Work out the finished part from the listing and answer in its coordinate system (mm). Face numbers are marked on the shaded views. A direction names the side the tool comes from. Give positions to 0.01 mm unless a question says otherwise; leave off trailing zeros. Order: outer loops, then holes, each group sorted by start corner. A loop starts at its lowest first (then second) coordinate and runs counter-clockwise, first axis right, second up. Notation, with made-up numbers: M 52.5,-16.5 L 63.5,-16.5 A29 cw 63.5,19.5 Z; hole C 3,35.25 d5. An arc over 180 degrees is marked long. One line per item, written item: value.
Solid Edge part; units mm, degrees
sketch "Sketch1" plane through (0, 0, 0) normal (0, -1, 0) x (1, 0, 0)
  line L0 (31.4924, 49.0939) -> (121.4924, 49.0939)
  line L1 (121.4924, 49.0939) -> (121.4924, 9.0939)
  line L2 (121.4924, 9.0939) -> (31.4924, 9.0939)
  line L3 (31.4924, 9.0939) -> (31.4924, 49.0939)
  dimension "D1" = 31.4924
  dimension "D2" = 121.4924
extrude "Protrusion1" add sketch "Sketch1" against normal blind 40
sketch "Sketch2" plane through (64.4924, 0, 22.0939) normal (0, -1, 0) x (1, 0, 0)
  line L0 (-18.0616, 9.8803) -> (-8, 10.7605)
  line L1 (-8, 10.7605) -> (-8, 18.0605)
  line L2 (-8, 18.0605) -> (34, 18.0605)
  line L3 (34, -4) -> (34, 18.0605)
  line L4 (-8, -4) -> (34, -4)
  line L5 (-8, -4) -> (-8, 3.3)
  line L6 (-8, 3.3) -> (-18.0616, 4.1803)
  line L7 (-18.0616, 4.1803) -> (-18.0616, 9.8803)
extrude "ExtrudedCutout_4" cut sketch "Sketch2" against normal blind 37
sketch "Sketch3" plane through (31.4924, 20, 22.0939) normal (-1, 0, 0) x (0, -1, 0)
  line L0 (-17, 2) -> (-17, 12)
  line L1 (-17, 12) -> (-10, 12)
  line L2 (-10, 12) -> (-10, 2)
  line L3 (-10, 2) -> (-17, 2)
  dimension "D1" = 17
  dimension "D2" = 17
  dimension "D3" = 10
extrude "Cutout1" cut sketch "Sketch3" against normal up to next
sketch "Sketch4" plane through (64.4924, 0, 22.0939) normal (0, -1, 0) x (1, 0, 0)
  line L0 (-8, 17.0605) -> (-18, 17.0605)
  line L1 (-18, 17.0605) -> (-18, -2.9395)
  line L2 (-18, -2.9395) -> (-8, -2.9395)
  line L3 (-8, -2.9395) -> (-8, 17.0605)
  line L4 (34, 17.0605) -> (44, 17.0605)
  line L5 (44, 17.0605) -> (44, -2.9395)
  line L6 (44, -2.9395) -> (34, -2.9395)
  line L7 (34, -2.9395) -> (34, 17.0605)
  dimension "D1" = 44
  dimension "D2" = 8
  dimension "D3" = 18
  dimension "D4" = 34
extrude "ExtrudedCutout_6" cut sketch "Sketch4" against normal blind 10
sketch "Sketch5" plane through (91.2324, 10, 21.645) normal (0, -1, 0) x (1, 0, 0)
  circle A0 centre (11.76, 12.5095) radius 1.65
  circle A1 centre (-39.24, 12.5095) radius 1.65
  circle A2 centre (-39.24, 2.5095) radius 1.65
  circle A3 centre (11.76, 2.5095) radius 1.65
  dimension "D1" = 39.24
  dimension "D2" = 11.76
  dimension "D3" = 39.24
extrude "Cutout2" cut sketch "Sketch5" against normal through all
sketch "Sketch6" plane through (68.9924, 0, 22.0939) normal (0, -1, 0) x (1, 0, 0)
  line L0 (-37.5, 27) -> (-37.5, -13)
  line L1 (-37.5, -13) -> (52.5, -13)
  line L2 (52.5, -13) -> (52.5, 27)
  line L3 (52.5, 27) -> (-37.5, 27)
  line L4 (-22.5616, 13.0605) -> (-22.5616, 18.0605)
  line L5 (-22.5616, 18.0605) -> (39.5, 18.0605)
  line L6 (39.5, 18.0605) -> (39.5, -4)
  line L7 (39.5, -4) -> (-22.5616, -4)
  line L8 (-22.5616, 13.0605) -> (-22.5616, -4)
  dimension "D1" = 39.5
extrude "ExtrudedProtrusion_4" add sketch "Sketch6" along normal blind 28.07
sketch "Sketch7" plane through (68.9924, -28.07, 22.0939) normal (0, -1, 0) x (1, 0, 0)
  circle A0 centre (-4.46, 7) radius 23.5
extrude "ExtrudedCutout_9" cut sketch "Sketch7" against normal blind 33.07
sketch "Sketch8" plane through (41.8429, -28.07, 29.0939) normal (0, -1, 0) x (0, 0, 1)
  line L0 (0, 10.3505) -> (5, 10.3505)
  line L1 (5, 10.3505) -> (5, -79.6495)
  line L2 (5, -79.6495) -> (0, -79.6495)
  line L3 (0, -79.6495) -> (-5, -79.6495)
  line L4 (-5, -79.6495) -> (-5, 10.3505)
  line L5 (-5, 10.3505) -> (0, 10.3505)
  dimension "D1" = 5
extrude "Cutout3" cut sketch "Sketch8" against normal blind 15
sketch "Sketch9" plane through (76.4924, 5.965, 49.0939) normal (0, 0, 1) x (-1, 0, 0)
  line L0 (-0.379, 0.965) -> (24.299, 0.965)
  line L1 (24.299, 0.965) -> (45, 0.965)
  line L2 (45, 0.965) -> (55, 0.965)
  line L3 (55, 0.965) -> (55, -9.035)
  line L4 (55, -9.035) -> (45, -9.035)
  line L5 (45, -9.035) -> (-45, -9.035)
  line L6 (-45, -9.035) -> (-55, -9.035)
  line L7 (-55, -9.035) -> (-55, 0.965)
  line L8 (-55, 0.965) -> (-45, 0.965)
  line L9 (-45, 0.965) -> (-0.379, 0.965)
  dimension "D1" = 55
  dimension "D2" = 45
  dimension "D3" = 45
  dimension "D4" = 55
extrude "ExtrudedProtrusion_9" add sketch "Sketch9" against normal blind 8
sketch "Sketch10" plane through (26.4924, 10, 41.0939) normal (0, 0, -1) x (-1, 0, 0)
  circle A0 centre (0, 0) radius 2
  circle A1 centre (-100, 0) radius 2
extrude "Cutout4" cut sketch "Sketch10" against normal through all
chamfer "Chamfer_1" distance 10 angle 45 1 edges at (31.4924, 15, 45.0939)
chamfer "Chamfer_2" distance 10 angle 45 1 edges at (31.4924, 5, 45.0939)
chamfer "Chamfer_3" distance 10 angle 45 1 edges at (121.4924, 15, 45.0939)
chamfer "Chamfer_4" distance 10 angle 45 1 edges at (121.4924, 5, 45.0939)
sketch "Sketch11" plane through (76.4924, 5.965, 49.0939) normal (0, 0, 1) x (1, 0, 0)
  line L0 (-55, 9.035) -> (55, 9.035)
  line L1 (55, 9.035) -> (45, 34.035)
  line L2 (45, 34.035) -> (-45, 34.035)
  line L3 (-45, 34.035) -> (-55, 9.035)
extrude "Cutout5" cut sketch "Sketch11" against normal through all
sketch "Sketch12" plane through (99.1819, -28.07, 41.5939) normal (0, -1, 0) x (1, 0, 0)
  line L0 (-58.1495, -12.5) -> (-58.1495, 7.5)
  line L1 (-58.1495, 7.5) -> (0, 7.5)
  line L2 (0, 7.5) -> (9.3829, 7.5)
  line L3 (9.3829, 7.5) -> (9.3829, -32.5)
  line L4 (-58.1495, -32.5) -> (9.3829, -32.5)
  line L5 (-58.1495, -12.5) -> (-58.1495, -32.5)
extrude "Cutout6" cut sketch "Sketch12" against normal up to vertex (33.07 mm away)
sketch "Sketch13" plane through (36.2624, -28.07, 41.5939) normal (0, -1, 0) x (0, 0, -1)
  line L0 (2.5, -4.77) -> (2.5, 4.77)
  line L1 (2.5, 4.77) -> (7.5, 4.77)
  line L2 (7.5, 4.77) -> (7.5, -4.77)
  line L3 (7.5, -4.77) -> (2.5, -4.77)
extrude "Cutout7" cut sketch "Sketch13" against normal up to vertex (15 mm away)
sketch "Sketch14" plane through (36.2624, -28.07, 41.5939) normal (0, -1, 0) x (0, 0, -1)
  line L0 (22.5, 4.77) -> (22.5, -4.77)
  line L1 (22.5, -4.77) -> (17.5, -4.77)
  line L2 (17.5, -4.77) -> (17.5, 4.77)
  line L3 (17.5, 4.77) -> (22.5, 4.77)
extrude "Cutout8" cut sketch "Sketch14" against normal up to vertex (15 mm away)
sketch "Sketch15" plane through (36.2624, -28.07, 41.5939) normal (0, -1, 0) x (0, 0, -1)
  line L0 (2.5, 85.23) -> (7.5, 85.23)
  line L1 (7.5, 85.23) -> (7.5, 72.3024)
  line L2 (2.5, 72.3024) -> (7.5, 72.3024)
  line L3 (2.5, 85.23) -> (2.5, 72.3024)
extrude "Cutout9" cut sketch "Sketch15" against normal up to vertex (15 mm away)
sketch "Sketch16" plane through (36.2624, -28.07, 41.5939) normal (0, -1, 0) x (0, 0, -1)
  line L0 (22.5, 85.23) -> (22.5, 72.3024)
  line L1 (22.5, 72.3024) -> (17.5, 72.3024)
  line L2 (17.5, 72.3024) -> (17.5, 85.23)
  line L3 (17.5, 85.23) -> (22.5, 85.23)
extrude "Cutout10" cut sketch "Sketch16" against normal up to vertex (15 mm away)
sketch "Sketch17" plane through (36.2624, -28.07, 44.0939) normal (0, -1, 0) x (1, 0, 0)
  line L0 (4.77, 5) -> (4.77, -5)
  line L1 (4.77, -5) -> (-4.77, -5)
  line L2 (-4.77, -5) -> (-4.77, 5)
  line L3 (-4.77, 5) -> (4.77, 5)
extrude "ExtrudedProtrusion_10" add sketch "Sketch17" along normal blind 4
sketch "Sketch18" plane through (36.2624, -28.07, 14.0939) normal (0, -1, 0) x (1, 0, 0)
  line L0 (85.23, 25) -> (85.23, 35)
  line L1 (85.23, 35) -> (72.3024, 35)
  line L2 (72.3024, 35) -> (72.3024, 25)
  line L3 (72.3024, 25) -> (85.23, 25)
extrude "Protrusion2" add sketch "Sketch18" along normal blind 4
sketch "Sketch19" plane through (36.2624, -28.07, 14.0939) normal (0, -1, 0) x (1, 0, 0)
  line L0 (72.3024, 5) -> (72.3024, -5)
  line L1 (72.3024, -5) -> (85.23, -5)
  line L2 (85.23, 5) -> (85.23, -5)
  line L3 (72.3024, 5) -> (85.23, 5)
extrude "Protrusion3" add sketch "Sketch19" along normal blind 4
sketch "Sketch20" plane through (36.2624, -28.07, 14.0939) normal (0, -1, 0) x (1, 0, 0)
  line L0 (-4.77, -5) -> (-4.77, 5)
  line L1 (-4.77, 5) -> (4.77, 5)
  line L2 (4.77, 5) -> (4.77, -5)
  line L3 (4.77, -5) -> (-4.77, -5)
extrude "Protrusion4" add sketch "Sketch20" along normal blind 4
sketch "Sketch21" plane through (36.2624, -32.07, 44.0939) normal (0, -1, 0) x (1, 0, 0)
  circle A0 centre (0, 0) radius 2.25
extrude "Cutout11" cut sketch "Sketch21" against normal blind 5
sketch "Sketch22" plane through (115.0286, -32.07, 14.0939) normal (0, -1, 0) x (1, 0, 0)
  circle A0 centre (1.4638, 0) radius 2.25
  dimension "D1" = 1.4638
  dimension "D2" = 1.4638
extrude "Cutout12" cut sketch "Sketch22" against normal blind 5
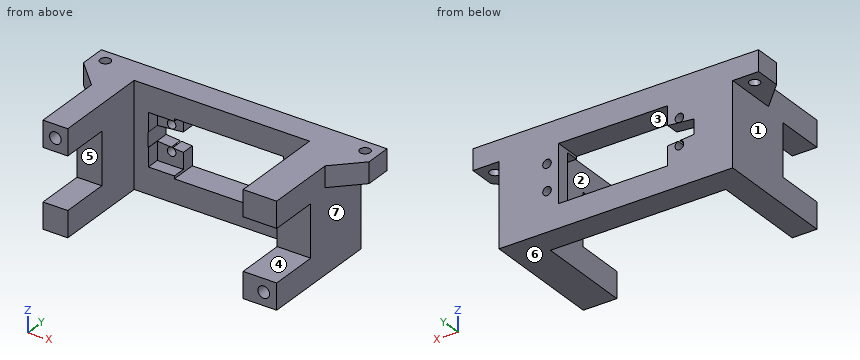
(1) Given P1, Ø5.5, axis at y = 7, z = 23, coming from the +X side; P2, Ø5, axis at y = -0.5, z = 31, coming from the -X side; P3, Ø8, axis at x = 51.5, z = 23, coming from the -Y side, each flat-ended and moving along its own axis, determine where each tip first touches the part or whether it passes through.
Findings:
P1: stops at x = 121.49
P2: stops at x = 31.49
P3: stops at y = 5
(2) Section A-A, the plane x = 86 is taken. Give the vertices of the cut face in (y, z).
Findings:
outline: M 5,9.09 L 15,9.09 L 15,18.09 L 5,18.09 Z; M 5,40.15 L 15,40.15 L 15,49.09 L 5,49.09 Z
(3) Section D-D, the plane y = -3 is taken. Give the vertices of the cut face in (x, z), then the cut area to 3 significant figures.
Findings:
outline: M 29.49,41.09 L 31.49,41.09 L 31.49,9.09 L 41.03,9.09 L 41.03,49.09 L 29.49,49.09 Z; M 108.56,9.09 L 121.49,9.09 L 121.49,41.09 L 123.49,41.09 L 123.49,49.09 L 108.56,49.09 Z
area: 931 mm^2
(4) Find the intervals of material crossed by probe 1 along X at (y, z) = (-13, 12); probe 2 along Z at (x, y) = (109.5, -15); probe 3 along X at (y, z) = (9.5, 23), in increasing order. Write a range as from..to.
Findings:
probe 1: x = 31.49..41.03, 108.56..121.49
probe 2: z = 9.09..19.09, 39.09..49.09
probe 3: x = 31.49..46.49, 108.49..121.49
(5) Determine the mould class of the marked faces 4, 5, 6 and 7 for opening direction Z: pulls with the +Z half, pulls with the -Z half, needs draft (parallel to the pull), parting line crosses it, or undercut.
Findings:
face 4: undercut
face 5: undercut
face 6: pulls with the -Z half
face 7: needs draft
(6) Which of the six approach directions +Z, -Z, +X, -X, +Y, -Y give full straight-line access (tool end or side, diameter ignored) to the marked faces 1, 2 and 3?
Findings:
face 1: -Z, -X, -Y
face 2: +Z, -Z, -Y
face 3: +Y, -Y
(7) Section B-B, the plane y = -12 is taken. Give the vertices of the cut face in (x, z), then the cut area to 3 significant figures.
Findings:
outline: M 31.49,9.09 L 41.03,9.09 L 41.03,49.09 L 31.49,49.09 Z; M 108.56,9.09 L 121.49,9.09 L 121.49,49.09 L 108.56,49.09 Z
area: 899 mm^2
(8) Section C-C, the plane y = -23.5 is taken. Give the vertices of the cut face in (x, z).
Findings:
outline: M 31.49,9.09 L 41.03,9.09 L 41.03,19.09 L 31.49,19.09 Z; M 31.49,39.09 L 41.03,39.09 L 41.03,49.09 L 31.49,49.09 Z; M 108.56,9.09 L 121.49,9.09 L 121.49,19.09 L 108.56,19.09 Z; M 108.56,39.09 L 121.49,39.09 L 121.49,49.09 L 108.56,49.09 Z
